Geometry: final body of the model. Coordinates: model frame, mm. A direction names the side the tool comes from. Round coordinates to 2 decimals unless told otherwise and drop trailing zeros. Loops run counter-clockwise (first coordinate to the right, second up) from the corner with the lowest first, then second, coordinate; pieces in that order, holes last. Notation, with made-up numbers: (30, -21) - (78, -21) arc R24 ccw to (78, 15) - close; hole circle Ø6 at (-39.5, -18.75). An arc over 180 degrees is marked (long way). Return JSON: item names as keys, results as strings. Group by question number.
1. Section B-B on x = -1. Return loops of the section in (y, z).
2. Material intervals for probe 1 along Y at (x, z) = (4.75, -2.25); probe 2 along Z at (x, y) = (-0.5, -14); probe 3 along Z at (x, y) = (2.25, -15.25), sorted ascending.
3. Set-up query: faces 1 (the face through (0, 0, 0)), 2 (the face through (0, -17.462, 8)), 3 (the face through (0, -11.112, 0)). Return all of +Z, -Z, +X, -X, +Y, -Y with unobstructed straight access to the full face (end or side cutting, diameter ignored); none if empty.
4. Draft query along X for faces 4 (the face through (1.588, -19, -8)), 5 (the face through (-6.5, -20.638, 0.1)). Return one class per face: +X half, -X half, draft (parallel to the pull), parting line (faces both ways), or undercut.
5. First-contact query: pin 1 Ø1.6 at (x, z) = (0.5, 7.5) entering from -Y; pin 2 Ø3 at (x, y) = (7, -8.5) entering from +Z; pin 3 Ø1 at (y, z) = (-8, 2.5) entering from +X. Flat tips, straight axial feed; report the tip coordinate or a pass-through.
6. Section C-C on z = 2.5. Return loops of the section in (x, y), and give its area (3 significant figures).
7. Section D-D on y = -3.5. Return loops of the section in (x, z) (3 decimals), and give its area (3 significant figures).
from build123d import *

# Parameters (mm, degrees)
F0_W     = 19.05
F0_H     = 19.05
F1_DEPTH = 20.6375
F2_R     = 6.35
F3_DEPTH = 9.525
F5_DEPTH = 25.4
F7_DEPTH = 25.4


with BuildPart() as f1:
    # F0 (on Front) → F1 (new body)
    with BuildSketch(Plane.XZ):
        Rectangle(F0_W, F0_H)
    extrude(amount=F1_DEPTH)

    # F2 (on face) → F3 (cut)
    with BuildSketch(Plane.XZ.offset(20.6375)):
        Circle(F2_R)
    extrude(amount=-F3_DEPTH, mode=Mode.SUBTRACT)

    # F4 (on face) → F5 (cut)
    with BuildSketch(Plane.XY.offset(9.525)):
        Polygon((-1.5875, -20.6375), (0, -20.6375), (1.5875, -20.6375), (1.5875, -17.4625), (-1.5875, -17.4625), align=None)
    extrude(amount=-F5_DEPTH, mode=Mode.SUBTRACT)

    # F6 (on face) → F7 (cut)
    with BuildSketch(Plane(origin=(0, 0, 0), x_dir=(-1, 0, 0), z_dir=(0, 1, 0))):
        with BuildLine():
            ThreePointArc((-9.525, 0), (-6.7351920908, 6.7351920908), (0, 9.525))
            Line((0, 9.525), (-9.525, 9.525))
            Line((-9.525, 9.525), (-9.525, 0))
        make_face()
        with BuildLine():
            ThreePointArc((0, 9.525), (6.7351920908, 6.7351920908), (9.525, 0))
            Line((9.525, 0), (9.525, 9.525))
            Line((9.525, 9.525), (0, 9.525))
        make_face()
        with BuildLine():
            Line((-9.525, -9.525), (0, -9.525))
            ThreePointArc((0, -9.525), (-6.7351920908, -6.7351920908), (-9.525, 0))
            Line((-9.525, 0), (-9.525, -9.525))
        make_face()
        with BuildLine():
            Line((9.525, -9.525), (9.525, 0))
            ThreePointArc((9.525, 0), (6.7351920908, -6.7351920908), (0, -9.525))
            Line((0, -9.525), (9.525, -9.525))
        make_face()
    extrude(amount=-F7_DEPTH, mode=Mode.SUBTRACT)


solid = f1.part
Taken from the geometry:
{
 "1": {"outline": "(-17.46, -9.47) - (0, -9.47) - (0, 9.47) - (-17.46, 9.47) - (-17.46, 6.27) - (-11.11, 6.27) - (-11.11, -6.27) - (-17.46, -6.27) - close"},
 "2": {"probe 1": "-11.11 to 0", "probe 2": "-9.51 to -6.33, 6.33 to 9.51", "probe 3": "-9.26 to -5.94, 5.94 to 9.26"},
 "3": {"face 1": "+Z, -Z, +X, -X, +Y", "face 2": "+Z, -Z, -Y", "face 3": "-Y"},
 "4": {"face 4": "undercut", "face 5": "draft"},
 "5": {"pin 1": "y = -17.46", "pin 2": "z = 7.78", "pin 3": "x = 9.31"},
 "6": {"outline": "(-9.19, -20.64) - (-5.84, -20.64) - (-5.84, -11.11) - (5.84, -11.11) - (5.84, -20.64) - (9.19, -20.64) - (9.19, 0) - (-9.19, 0) - close", "area": "268 mm2"},
 "7": {"outline": "circle Ø19.05 at (0, 0)", "area": "285 mm2"}
}
